from build123d import *

# Parameters (mm, degrees)
SKETCH1_W            = 1044
SKETCH1_H            = 348
BOSS_EXTRUDE1_DEPTH  = 321.9
CHAMFER2_SIZE        = 222
CHAMFER2_SIZE2       = 103.52030011
FILLET1_R            = 100
SCALE1_SCALE         = 0.115
SKETCH175_W          = 20
SKETCH175_H          = 12
BOSS_EXTRUDE12_DEPTH = 25
SKETCH176_W          = 5
SKETCH176_H          = 25
CUT_EXTRUDE1_DEPTH   = 30
SKETCH177_R          = 2.25
CUT_EXTRUDE2_DEPTH   = 30
CUT_EXTRUDE4_DEPTH   = 25


with BuildPart() as part:
    # Sketch1 → Boss-Extrude1 (new body)
    with BuildSketch(Plane(origin=(0, 0, 0), x_dir=(1, 0, 0), z_dir=(0, 1, 0))):
        Rectangle(SKETCH1_W, SKETCH1_H)
    extrude(amount=BOSS_EXTRUDE1_DEPTH)

    # Chamfer2
    chamfer2_edges = [part.edges().sort_by_distance(p)[0] for p in [
        (522, 321.9, 0),
    ]]
    chamfer2_side = [part.faces().sort_by_distance(p)[0] for p in [
        (0, 321.9, 0),
    ]]
    chamfer(chamfer2_edges, length=CHAMFER2_SIZE, length2=CHAMFER2_SIZE2, reference=chamfer2_side[0])

    # Fillet1
    fillet1_edges = [part.edges().sort_by_distance(p)[0] for p in [
        (-522, 321.9, 0),
        (-522, 0, 0),
        (-522, 160.95, -174),
        (-522, 160.95, 174),
    ]]
    fillet(fillet1_edges, radius=FILLET1_R)


with BuildPart() as part_1:
    # Scale1: scaled about (-4.978902211, 156.372589253, 0)
    add(part.part.scale(SCALE1_SCALE).moved(Location((-4.406328457, 138.389741489, 0))))


with BuildPart() as boss_extrude12_tool:
    # Sketch175 → Boss-Extrude12 (new body)
    with BuildSketch(Plane.XZ.offset(-138.389734505)):
        with Locations((-4.405349795, 0)):
            Rectangle(SKETCH175_W, SKETCH175_H)
    extrude(amount=BOSS_EXTRUDE12_DEPTH)


with BuildPart() as part_2:
    add(part_1.part)


with BuildPart() as part_3:
    # Boss-Extrude12: joined with boss_extrude12_tool
    add(part_2.part.fuse(boss_extrude12_tool.part, tol=0.00001))

    # Sketch176 → Cut-Extrude1 (cut)
    with BuildSketch(Plane(origin=(5.594650205, 0, 0), x_dir=(0, 0, -1), z_dir=(1, 0, 0))):
        with Locations((0, 125.889734505)):
            Rectangle(SKETCH176_W, SKETCH176_H)
    extrude(amount=-CUT_EXTRUDE1_DEPTH, mode=Mode.SUBTRACT)

    # Sketch177 → Cut-Extrude2 (cut)
    with BuildSketch(Plane(origin=(0, 0, -6), x_dir=(-1, 0, 0), z_dir=(0, 0, -1))):
        with Locations((4.405349795, 121.389734505)):
            Circle(SKETCH177_R)
    extrude(amount=-CUT_EXTRUDE2_DEPTH, mode=Mode.SUBTRACT)

    # Sketch179 → Cut-Extrude4 (cut)
    with BuildSketch(Plane.XZ.offset(-113.389734505)):
        Polygon((-14.405349795, 6), (20.594650205, 3.552561582), (20.594650205, -3.552561582), (-14.405349795, -6), (23.594650205, -6), (23.594650205, 6), align=None)
    extrude(amount=-CUT_EXTRUDE4_DEPTH, mode=Mode.SUBTRACT)


solid = part_3.part
Verification items for the finished model (mm, model axes). A direction names the side the tool comes from. Coordinates: 2 decimals unless noted, no trailing zeros. Order: outer loops, then holes, each group sorted by start corner. A loop starts at its lowest first (then second) coordinate and runs counter-clockwise, first axis right, second up. Notation, with made-up numbers: (-24.75, -39) -> (-18.75, -39) arc R25 ccw to (-18.75, -3) -> close; hole circle Ø11 at (2.25, 81.5). An arc over 180 degrees is marked (long way). Put each result on its own line as item: value. Start each with the question number.
1. Access from +Z, -Z, +X, -X, +Y, -Y to the whole of each face (thin tool, end or side, straight path). Record for faces 5 (the flat face through (-4, 126, 2.5)), 6 (the flat face through (-14.405, 126, 4)), 7 (the flat face through (-4.27, 125.71, -5.29)), 8 (the flat face through (-4.55, 125.71, 5.31)).
2. Material ranges on L1, parallel to Y at x = -33, z = 10; L2, parallel to X at y = 136, z = 3.5; L3, parallel to Z at x = -8.5, y = 131, recorded low to high. Write a range as [from, to].
3. Cross-section at A-A, the plane y = 136. Record the boundary of the cut face in (x, z).
4. Cross-section at C-C, the plane x = -1. Record the boundary of the cut face in (y, z).
5. Go/stop test with flat-tipped pins: pin 1 Ø1.5 at (x, z) = (43.5, 10.5) entering from -Y; pin 2 Ø2.5 at (x, y) = (-4.41, 121.39) entering from +Z; pin 3 Ø8 at (y, z) = (126.5, 1.5) entering from +X; pin 4 Ø6 at (x, y) = (-5, 130) entering from -Z. Record where each tip stops, or that it passes through.
6. Cross-section at D-D, the plane y = 166. Record the boundary of the cut face in (x, z), then the cut area to 3 significant figures.
7. Cross-section at B-B, the plane z = 1. Record the boundary of the cut face in (x, y).
8. Mould release check, pull along X, two halves, no side actions. Record for faces 1 (the flat face through (-14.405, 126, -4)), 2 (the cylindrical face through (-6.55, 122.07, -4)), 3 (the cylindrical face through (-6.55, 122.07, 3.96)), 4 (the flat face through (-12, 175.408, 0)): released by +X, released by -X, zero draft, split by the parting line, or undercut.
Computed:
1. face 5: +X, -X, -Y
1. face 6: +Z, -Z, -X, -Y
1. face 7: -Z, +X, -Y
1. face 8: +Z, +X, -Y
2. L1: [138.39, 175.41]
2. L2: [-14.41, 5.59]
2. L3: [-5.59, -2.5], [2.5, 5.59]
3. outline: (-14.41, -6) -> (5.59, -4.6) -> (5.59, -2.5) -> (-14.41, -2.5) -> close; (-14.41, 2.5) -> (5.59, 2.5) -> (5.59, 4.6) -> (-14.41, 6) -> close
4. outline: (113.39, -5.06) -> (138.39, -5.06) -> (138.39, -20.01) -> (175.41, -20.01) -> (175.41, 20.01) -> (138.39, 20.01) -> (138.39, 5.06) -> (113.39, 5.06) -> (113.39, 2.5) -> (138.39, 2.5) -> (138.39, -2.5) -> (113.39, -2.5) -> close
5. pin 1: y = 138.39
5. pin 2: through
5. pin 3: x = 5.59
5. pin 4: z = -5.55
6. outline: (-64.24, -10.6) arc R11.5 ccw to (-52.94, -20.01) -> (50.27, -20.01) -> (50.27, 20.01) -> (-52.94, 20.01) arc R11.5 ccw to (-64.24, 10.6) -> close
6. area: 4,530 mm2
7. outline: (-64.44, 149.89) arc R11.5 ccw to (-52.94, 138.39) -> (5.59, 138.39) -> (55.62, 138.39) -> (55.62, 163.5) -> (30.09, 175.41) -> (-52.94, 175.41) arc R11.5 ccw to (-64.44, 163.91) -> close
8. face 1: released by -X
8. face 2: undercut
8. face 3: undercut
8. face 4: zero draft
